Geometry: see drawing. Coordinates: mm, zero at the bounding-box minimum. Give positions to 0.01 mm unless a question says otherwise; leave off trailing zeros. Write each loop counter-clockwise with the first axis right and the second up, starting at its lowest first coordinate (ties: lowest second). Pieces come first, ordered by that corner, then holes. Notation, with made-up numbers: (23, 47) - (67, 47) arc R30 ccw to (67, 74) - close; hole circle Ø4 at (84.25, 76.5). An arc over 180 degrees is marked (long way). Use a Markdown table: item, result. Add a question column.
1. Material intervals for probe 1 along X at (y, z) = (7, 15); probe 2 along Z at (x, y) = (130, 4.5); probe 3 along X at (y, z) = (3.5, 11.75), sorted ascending.
2. Mould query, pull axis X, two halves, no side actions, for the marked faces 1, 2 and 3. Classes: released by +X, released by -X, zero draft, split by the parting line, or undercut.
3. Section query B-B, the plane y = 4.25. Return loops of the section in (x, z).
4. Section query D-D, the plane x = 70. Return loops of the section in (y, z) (3 decimals), plus the area to 3 significant figures.
5. Section query A-A, the plane x = 10. Return loops of the section in (y, z).
6. Section query C-C, the plane z = 15. Return loops of the section in (x, y) (3 decimals), plus the area to 3 significant figures.
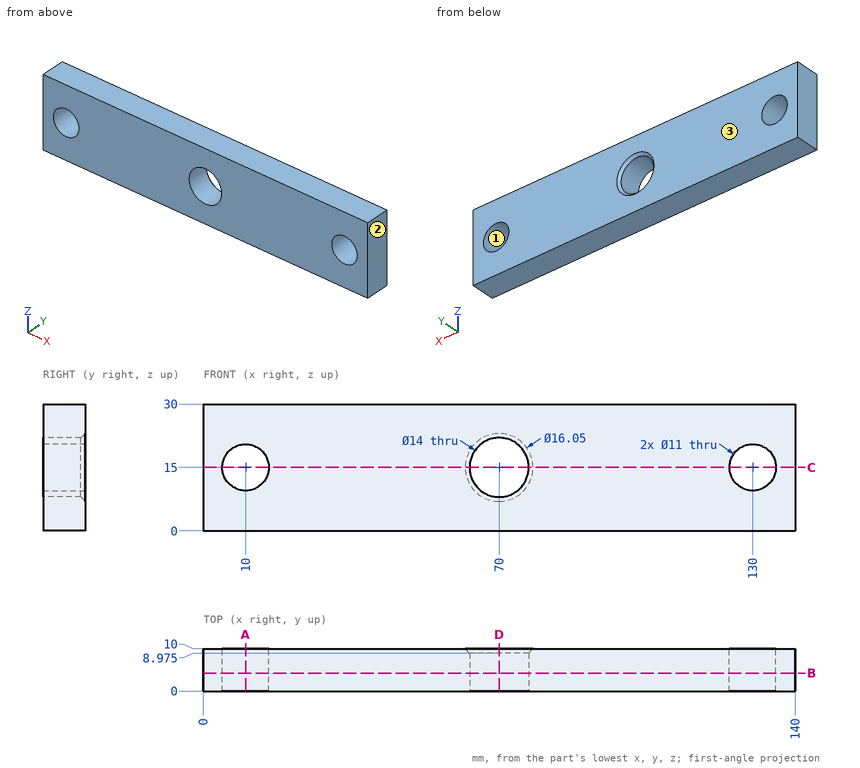
Result sheet:
| question | item | result |
|---|---|---|
| 1 | probe 1 | x = 0 to 4.5, 15.5 to 63, 77 to 124.5, 135.5 to 140 |
| 1 | probe 2 | z = 0 to 9.5, 20.5 to 30 |
| 1 | probe 3 | x = 0 to 5.56, 14.44 to 63.8, 76.2 to 125.56, 134.44 to 140 |
| 2 | face 1 | undercut |
| 2 | face 2 | released by +X |
| 2 | face 3 | zero draft |
| 3 | outline | (0, 0) - (140, 0) - (140, 30) - (0, 30) - close; hole circle Ø11 at (10, 15); hole circle Ø14 at (70, 15); hole circle Ø11 at (130, 15) |
| 4 | outline | (0, 0) - (10, 0) - (10, 6.975) - (8.975, 8) - (0, 8) - close; (0, 22) - (8.975, 22) - (10, 23.025) - (10, 30) - (0, 30) - close |
| 4 | area | 159 mm² |
| 5 | outline | (0, 0) - (10, 0) - (10, 9.5) - (0, 9.5) - close; (0, 20.5) - (10, 20.5) - (10, 30) - (0, 30) - close |
| 6 | outline | (0, 0) - (4.5, 0) - (4.5, 10) - (0, 10) - close; (15.5, 0) - (63, 0) - (63, 8.975) - (61.975, 10) - (15.5, 10) - close; (77, 0) - (124.5, 0) - (124.5, 10) - (78.025, 10) - (77, 8.975) - close; (135.5, 0) - (140, 0) - (140, 10) - (135.5, 10) - close |
| 6 | area | 1,040 mm² |
